from build123d import *

# Parameters (mm, degrees)
F0_R     = 10
F1_DEPTH = 4
F2_R     = 2
F3_W     = 4
F3_H     = 4
F4_DEPTH = 0.5
F5_SIZE  = 1.99999


# Not quite as in the source:
# - a fillet or chamfer is up to 0.001 mm smaller than in the source, because OpenCascade refuses the exact size


with BuildPart() as f1:
    # F0 (on Top) → F1 (new body)
    with BuildSketch(Plane.XY):
        with BuildLine():
            Line((50, 22.5), (50, 17.5))
            Line((50, 17.5), (0, 17.5))
            Line((0, 17.5), (-50, 0))
            ThreePointArc((-50, 0), (-40.9417194223, -12.6556443707), (-26.1515199646, -17.5))
            Line((-26.1515199646, -17.5), (50, -17.5))
            Line((50, -17.5), (50, -22.5))
            Line((50, -22.5), (55, -22.5))
            ThreePointArc((55, -22.5), (56.5936558821, -15.0125045804), (62.1990375221, -9.7988663689))
            ThreePointArc((62.1990375221, -9.7988663689), (98.7587484272, -9.3015269429), (135, -14.1421356237))
            ThreePointArc((135, -14.1421356237), (155, 0), (135, 14.1421356237))
            ThreePointArc((135, 14.1421356237), (98.7587484272, 9.3015269429), (62.1990375221, 9.7988663689))
            ThreePointArc((62.1990375221, 9.7988663689), (56.5936558821, 15.0125045804), (55, 22.5))
            Line((55, 22.5), (50, 22.5))
        make_face()
        with BuildLine():
            ThreePointArc((62.1990375221, -4.8343795659), (60.2509894701, 0), (62.1990375221, 4.8343795659))
            ThreePointArc((62.1990375221, 4.8343795659), (94.7590329876, 4.3577585856), (127.1470964452, 7.7332315503))
            ThreePointArc((127.1470964452, 7.7332315503), (125, 0), (127.1470964452, -7.7332315503))
            ThreePointArc((127.1470964452, -7.7332315503), (94.7590329876, -4.3577585856), (62.1990375221, -4.8343795659))
        make_face(mode=Mode.SUBTRACT)
        with Locations((140, 0)):
            Circle(F0_R, mode=Mode.SUBTRACT)
    extrude(amount=F1_DEPTH)

    # F2
    f2_edges = [f1.edges().sort_by_distance(p)[0] for p in [
        (127.147096, 7.733232, 2),
        (127.147096, -7.733232, 2),
    ]]
    fillet(f2_edges, radius=F2_R)

    # F3 (on face) → F4 (join)
    with BuildSketch(Plane.XZ.offset(17.5)):
        with Locations((48, 2)):
            Rectangle(F3_W, F3_H)
    extrude(amount=F4_DEPTH)

    # F5 (size 2 in the source; OpenCascade refuses exactly that, so slightly less here)
    f5_edges = [f1.edges().sort_by_distance(p)[0] for p in [
        (9.92424, -17.5, 4),
        (9.92424, -17.5, 0),
    ]]
    chamfer(f5_edges, length=F5_SIZE)


solid = f1.part
Input: part model. Units: mm. Frame: model coordinates. A direction names the side the tool comes from. Round coordinates to 2 decimals unless told otherwise and drop trailing zeros. Order: outer loops, then holes, each group sorted by start corner. A loop starts at its lowest first (then second) coordinate and runs counter-clockwise, first axis right, second up.
1. Cut plane B-B, the plane x = 94. Output: boundary loops of the cut face in (y, z).
The answers:
outline: (-9.06, 0) - (-4.32, 0) - (-4.32, 4) - (-9.06, 4) - close; (4.32, 0) - (9.06, 0) - (9.06, 4) - (4.32, 4) - close
2. Set-up query: faces 1 (the face through (98.25, -9.27, 1.97)), 2 (the face through (93.4, -4.3, 2)), 3 (the face through (25, 17.5, 2)), 4 (the face through (48, -18, 2)). Return all of +Z, -Z, +X, -X, +Y, -Y with unobstructed straight access to the full face (end or side cutting, diameter ignored); none if empty.
The answers:
face 1: +Z, -Z, -Y
face 2: +Z, -Z
face 3: +Z, -Z, -X, +Y
face 4: +Z, -Z, -X, -Y
3. Cut plane A-A, the plane x = 140. Output: boundary loops of the cut face in (y, z).
The answers:
outline: (-15, 0) - (-10, 0) - (-10, 4) - (-15, 4) - close; (10, 0) - (15, 0) - (15, 4) - (10, 4) - close
4. Cut plane C-C, the plane z = 1.1. State how many separate pieces and enclosed holes the cut face has, then the cut area to 3 significant figures.
The answers:
separate pieces: 1
enclosed holes: 2
area: 4,310 mm2
5. Mould query, pull axis Y, two halves, no side actions, for faces 5 (the face through (92.49, 4.266, 1.972)), 6 (the face through (50, -20, 2)), 7 (the face through (53, 22.5, 2)). Classes: released by +Y, released by -Y, zero draft, split by the parting line, or undercut.
The answers:
face 5: undercut
face 6: zero draft
face 7: released by +Y
6. Material intervals for line 1 (Y direction, x = 140, z = 1.35); line 2 (X direction, y = -3.5, z = 2.3); line 3 (X direction, y = -20, z = 2.4), sorted ascending.
The answers:
line 1: y = -15 to -10, 10 to 15
line 2: x = -48.27 to 61.19, 125.41 to 130.63, 149.37 to 154.59
line 3: x = 50 to 55.01
7. Pin query (flat end, axial travel): P1, Ø1.2, axis at x = 17.5, z = 2, coming from the +Y side; P2, Ø1.2, axis at x = 47, z = 2, coming from the -Y side. Return the tip coordinate at first contact, or that it passes through.
The answers:
P1: stops at y = 17.5
P2: stops at y = -18
